Input: part model. Units: mm. Frame: model coordinates. A direction names the side the tool comes from. Give positions to 0.01 mm unless a question says otherwise; leave off trailing zeros. Loops run counter-clockwise (first coordinate to the right, second up) from the corner with the lowest first, then second, coordinate; pieces in that order, holes last. Notation, with made-up numbers: (23.25, 44.5) - (57.25, 44.5) arc R24 ccw to (57.25, 77.5) - close; hole circle Ø4 at (29.25, 19.5). An arc over 180 degrees is marked (long way). Answer as a JSON object with one key per item and string values. Group by question number.
(1) Pin query (flat end, axial travel): P1, Ø14, axis at x = 38, y = 0, coming from the +Z side; P2, Ø2, axis at x = 15.5, y = -2.5, coming from the -Z side; P3, Ø14, axis at x = 19, y = -32.91, coming from the +Z side; P4, Ø3, axis at x = -3, y = 34.5, coming from the +Z side. Return the tip coordinate at first contact, or that it passes through.
(2) Section query B-B (x = 19). Return loops of the section in (y, z).
(3) Material intervals for L1, parallel to Y at x = 38, z = 35; L2, parallel to X at y = 0, z = 17; L3, parallel to Y at x = 19, z = 8, sorted ascending.
(4) Section query C-C (z = 7). Return loops of the section in (x, y).
(5) Section query A-A (x = -42). Return loops of the section in (y, z).
(6) Mould query, pull axis Y, two halves, no side actions, for faces 4 (the flat face through (12.3, 22.6, 20)), 5 (the flat face through (24, -38, 10)), 6 (the cylindrical face through (-16.231, 27.586, 23.752)), 7 (the flat face through (-24.65, 43.503, 10.14)). Classes: +Y half, -Y half, draft (parallel to the pull), parting line (faces both ways), or undercut.
(7) Access query for faces 1 (the flat face through (-44, -12, 15)), 2 (the flat face through (18, -20, 20)), 3 (the flat face through (27, 12, 35)). Directions: +Z, -Z, +X, -X, +Y, -Y. A direction counts if a zero-diameter tool reaches every point of the face in a straight line with its end or side. Return the directions, or none.
(8) Section query D-D (y = -10). Return loops of the section in (x, z).
```python
from build123d import *

# Parameters (mm, degrees)
F1_R            = 6
F2_DEPTH        = 20
F3_DEPTH        = 30
F3_DEPTH_BACK   = 20
F4_DEPTH        = 10
F6_DEPTH        = 12.5
F6_COPIES_COUNT = 3


# Not quite as in the source:
# - a pattern or mirror of a feature is missing from the dataset's text; its kind, count and spacing are read off the source's solid


with BuildPart() as f2:
    # F1 (on offset) → F2 (new body, through all)
    with BuildSketch(Plane.XY.offset(20)):
        with BuildLine():
            ThreePointArc((-29.3923048454, 26.9089653438), (-30.5911098969, 36.0147939544), (-24.9999998757, 43.301270261))
            Line((-24.9999998757, 43.301270261), (-50, 28.8675134595))
            Line((-50, 28.8675134595), (-50, 12))
            Line((-50, 12), (-38, 12))
            ThreePointArc((-38, 12), (-26, 0), (-38, -12))
            Line((-38, -12), (-50, -12))
            Line((-50, -12), (-50, -28.8675134595))
            Line((-50, -28.8675134595), (-24.9999998757, -43.301270261))
            ThreePointArc((-24.9999998757, -43.301270261), (-30.5911098969, -36.0147939544), (-29.3923048454, -26.9089653438))
            Line((-29.3923048454, -26.9089653438), (-22.8923048454, -15.6506350946))
            Line((-22.8923048454, -15.6506350946), (-18.3923048454, -7.8564064606))
            ThreePointArc((-18.3923048454, -7.8564064606), (-20, 0), (-18.3923048454, 7.8564064606))
            Line((-18.3923048454, 7.8564064606), (-22.8923048454, 15.6506350946))
            Line((-22.8923048454, 15.6506350946), (-29.3923048454, 26.9089653438))
        make_face()
        with BuildLine():
            Line((-38, 12), (-50, 12))
            Line((-50, 12), (-50, -12))
            Line((-50, -12), (-38, -12))
            ThreePointArc((-38, -12), (-26, 0), (-38, 12))
        make_face()
        with Locations((-38, 0)):
            Circle(F1_R, mode=Mode.SUBTRACT)
    extrude(amount=-F2_DEPTH)



with BuildPart() as f2b:
    # F1 (on offset) → F2, piece 2 (new body, through all)
    with BuildSketch(Plane.XY.offset(20)):
        with BuildLine():
            Line((50, -28.8675134595), (50, 0))
            ThreePointArc((50, 0), (46.4852813742, -8.4852813742), (38, -12))
            Line((38, -12), (25, -12))
            Line((25, -12), (16, -12))
            ThreePointArc((16, -12), (10, -17.3205080757), (2.3923048454, -19.8564064606))
            Line((2.3923048454, -19.8564064606), (-2.1076951546, -27.6506350946))
            Line((-2.1076951546, -27.6506350946), (-8.6076951546, -38.9089653438))
            ThreePointArc((-8.6076951546, -38.9089653438), (-15.8941713895, -44.5000752407), (-24.9999998757, -43.301270261))
            Line((-24.9999998757, -43.301270261), (0, -57.735026919))
            Line((0, -57.735026919), (14.6076951546, -49.3012701892))
            Line((14.6076951546, -49.3012701892), (8.6076951546, -38.9089653438))
            ThreePointArc((8.6076951546, -38.9089653438), (13, -22.5166604984), (29.3923048454, -26.9089653438))
            Line((29.3923048454, -26.9089653438), (35.3923048454, -37.3012701892))
            Line((35.3923048454, -37.3012701892), (50, -28.8675134595))
        make_face()
        with BuildLine():
            Line((14.6076951546, -49.3012701892), (35.3923048454, -37.3012701892))
            Line((35.3923048454, -37.3012701892), (29.3923048454, -26.9089653438))
            ThreePointArc((29.3923048454, -26.9089653438), (13, -22.5166604984), (8.6076951546, -38.9089653438))
            Line((8.6076951546, -38.9089653438), (14.6076951546, -49.3012701892))
        make_face()
        with Locations((19, -32.9089653438)):
            Circle(F1_R, mode=Mode.SUBTRACT)
    extrude(amount=-F2_DEPTH)


with BuildPart() as f2c:
    # F1 (on offset) → F2, piece 3 (new body, through all)
    with BuildSketch(Plane.XY.offset(20)):
        with BuildLine():
            Line((50, 0), (50, 28.8675134595))
            Line((50, 28.8675134595), (35.3923048454, 37.3012701892))
            Line((35.3923048454, 37.3012701892), (29.3923048454, 26.9089653438))
            ThreePointArc((29.3923048454, 26.9089653438), (13, 22.5166604984), (8.6076951546, 38.9089653438))
            Line((8.6076951546, 38.9089653438), (14.6076951546, 49.3012701892))
            Line((14.6076951546, 49.3012701892), (0, 57.735026919))
            Line((0, 57.735026919), (-24.9999998757, 43.301270261))
            ThreePointArc((-24.9999998757, 43.301270261), (-15.8941713895, 44.5000752407), (-8.6076951546, 38.9089653438))
            Line((-8.6076951546, 38.9089653438), (-2.1076951546, 27.6506350946))
            Line((-2.1076951546, 27.6506350946), (2.3923048454, 19.8564064606))
            ThreePointArc((2.3923048454, 19.8564064606), (10, 17.3205080757), (16, 12))
            Line((16, 12), (25, 12))
            Line((25, 12), (38, 12))
            ThreePointArc((38, 12), (46.4852813742, 8.4852813742), (50, 0))
        make_face()
        with BuildLine():
            Line((29.3923048454, 26.9089653438), (35.3923048454, 37.3012701892))
            Line((35.3923048454, 37.3012701892), (14.6076951546, 49.3012701892))
            Line((14.6076951546, 49.3012701892), (8.6076951546, 38.9089653438))
            ThreePointArc((8.6076951546, 38.9089653438), (13, 22.5166604984), (29.3923048454, 26.9089653438))
        make_face()
        with Locations((19, 32.9089653438)):
            Circle(F1_R, mode=Mode.SUBTRACT)
    extrude(amount=-F2_DEPTH)


with BuildPart() as f2_1:
    add(f2.part)

    add(f2b.part)  # F3 merges F2b

    add(f2c.part)  # F3 merges F2c
    # F1 (on offset) → F3 (join, two sides)
    with BuildSketch(Plane.XY.offset(20)) as f3_sk:
        with BuildLine():
            ThreePointArc((-8.6076951546, 38.9089653438), (-15.8941713895, 44.5000752407), (-24.9999998757, 43.301270261))
            ThreePointArc((-24.9999998757, 43.301270261), (-30.5911098969, 36.0147939544), (-29.3923048454, 26.9089653438))
            Line((-29.3923048454, 26.9089653438), (-22.8923048454, 15.6506350946))
            Line((-22.8923048454, 15.6506350946), (-2.1076951546, 27.6506350946))
            Line((-2.1076951546, 27.6506350946), (-8.6076951546, 38.9089653438))
        make_face()
        with Locations((-19, 32.9089653438)):
            Circle(F1_R, mode=Mode.SUBTRACT)
        with BuildLine():
            Line((16, -12), (25, -12))
            Line((25, -12), (25, 12))
            Line((25, 12), (16, 12))
            ThreePointArc((16, 12), (10, 17.3205080757), (2.3923048454, 19.8564064606))
            Line((2.3923048454, 19.8564064606), (-2.1076951546, 27.6506350946))
            Line((-2.1076951546, 27.6506350946), (-22.8923048454, 15.6506350946))
            Line((-22.8923048454, 15.6506350946), (-18.3923048454, 7.8564064606))
            ThreePointArc((-18.3923048454, 7.8564064606), (-20, 0), (-18.3923048454, -7.8564064606))
            Line((-18.3923048454, -7.8564064606), (-22.8923048454, -15.6506350946))
            Line((-22.8923048454, -15.6506350946), (-2.1076951546, -27.6506350946))
            Line((-2.1076951546, -27.6506350946), (2.3923048454, -19.8564064606))
            ThreePointArc((2.3923048454, -19.8564064606), (10, -17.3205080757), (16, -12))
        make_face()
        with BuildLine():
            ThreePointArc((38, -12), (46.4852813742, -8.4852813742), (50, 0))
            ThreePointArc((50, 0), (46.4852813742, 8.4852813742), (38, 12))
            Line((38, 12), (25, 12))
            Line((25, 12), (25, -12))
            Line((25, -12), (38, -12))
        make_face()
        with Locations((38, 0)):
            Circle(F1_R, mode=Mode.SUBTRACT)
        with BuildLine():
            ThreePointArc((-29.3923048454, -26.9089653438), (-30.5911098969, -36.0147939544), (-24.9999998757, -43.301270261))
            ThreePointArc((-24.9999998757, -43.301270261), (-15.8941713895, -44.5000752407), (-8.6076951546, -38.9089653438))
            Line((-8.6076951546, -38.9089653438), (-2.1076951546, -27.6506350946))
            Line((-2.1076951546, -27.6506350946), (-22.8923048454, -15.6506350946))
            Line((-22.8923048454, -15.6506350946), (-29.3923048454, -26.9089653438))
        make_face()
        with Locations((-19, -32.9089653438)):
            Circle(F1_R, mode=Mode.SUBTRACT)
    extrude(amount=F3_DEPTH)
    extrude(f3_sk.sketch, amount=-F3_DEPTH_BACK)

    # F1 (on offset) → F4 (cut)
    with BuildSketch(Plane.XY.offset(20)):
        with BuildLine():
            Line((-38, 12), (-50, 12))
            Line((-50, 12), (-50, -12))
            Line((-50, -12), (-38, -12))
            ThreePointArc((-38, -12), (-26, 0), (-38, 12))
        make_face()
        with Locations((-38, 0)):
            Circle(F1_R, mode=Mode.SUBTRACT)
        with BuildLine():
            Line((14.6076951546, -49.3012701892), (35.3923048454, -37.3012701892))
            Line((35.3923048454, -37.3012701892), (29.3923048454, -26.9089653438))
            ThreePointArc((29.3923048454, -26.9089653438), (13, -22.5166604984), (8.6076951546, -38.9089653438))
            Line((8.6076951546, -38.9089653438), (14.6076951546, -49.3012701892))
        make_face()
        with Locations((19, -32.9089653438)):
            Circle(F1_R, mode=Mode.SUBTRACT)
        with BuildLine():
            Line((29.3923048454, 26.9089653438), (35.3923048454, 37.3012701892))
            Line((35.3923048454, 37.3012701892), (14.6076951546, 49.3012701892))
            Line((14.6076951546, 49.3012701892), (8.6076951546, 38.9089653438))
            ThreePointArc((8.6076951546, 38.9089653438), (13, 22.5166604984), (29.3923048454, 26.9089653438))
        make_face()
        with Locations((19, 32.9089653438)):
            Circle(F1_R, mode=Mode.SUBTRACT)
    extrude(amount=-F4_DEPTH, mode=Mode.SUBTRACT)

    # F5 (on Front) → F6 (cut, symmetric)
    with BuildSketch(Plane.XZ):
        Polygon((50, 50), (25, 50), (50, 38.3423085461), align=None)
    f6 = extrude(amount=F6_DEPTH, both=True, mode=Mode.SUBTRACT)

    # F6_copies: F6 ×3 about axis
    f6_copies_axis = Axis((0, 0, 0), (0, 0, 1))
    for i in range(1, F6_COPIES_COUNT):
        add(f6.rotate(f6_copies_axis, i * 360 / F6_COPIES_COUNT), mode=Mode.SUBTRACT)


solid = f2_1.part
```
Recorded:
{
 "1": {"P1": "stops at z = 47.2", "P2": "stops at z = 0", "P3": "stops at z = 10", "P4": "stops at z = 20"},
 "2": {"outline": "(-46.77, 0) - (-38.91, 0) - (-38.91, 10) - (-46.77, 10) - close; (-26.91, 0) - (26.91, 0) - (26.91, 10) - (20.91, 10) - (20.91, 20) - (12, 20) - (12, 50) - (-12, 50) - (-12, 20) - (-20.91, 20) - (-20.91, 10) - (-26.91, 10) - close; (38.91, 0) - (46.77, 0) - (46.77, 10) - (38.91, 10) - close"},
 "3": {"L1": "y = -12 to -6, 6 to 12", "L2": "x = -26 to 32, 44 to 50", "L3": "y = -46.77 to -38.91, -26.91 to 26.91, 38.91 to 46.77"},
 "4": {"outline": "(-50, -28.87) - (0, -57.74) - (50, -28.87) - (50, 28.87) - (0, 57.74) - (-50, 28.87) - close; hole circle Ø12 at (-38, 0); hole circle Ø12 at (-19, -32.91); hole circle Ø12 at (-19, 32.91); hole circle Ø12 at (19, -32.91); hole circle Ø12 at (19, 32.91); hole circle Ø12 at (38, 0)"},
 "5": {"outline": "(-33.49, 0) - (-4.47, 0) - (-4.47, 10) - (-12, 10) - (-12, 20) - (-33.49, 20) - close; (4.47, 0) - (33.49, 0) - (33.49, 20) - (12, 20) - (12, 10) - (4.47, 10) - close"},
 "6": {"face 4": "draft", "face 5": "undercut", "face 6": "undercut", "face 7": "+Y half"},
 "7": {"face 1": "+Z, -X", "face 2": "+Z, +X, -Y", "face 3": "+Z, +X, +Y"},
 "8": {"outline": "(-50, 0) - (50, 0) - (50, 20) - (44.63, 20) - (44.63, 40.84) - (25, 50) - (-19.63, 50) - (-19.63, 20) - (-31.37, 20) - (-31.37, 10) - (-50, 10) - close"}
}
